For this review, take the finished solid that the model builds, in its own axes (mm). Face numbers are marked on the shaded views. A direction names the side the tool comes from. Give positions to 0.01 mm unless a question says otherwise; leave off trailing zeros. Write each loop counter-clockwise with the first axis right and the second up, starting at its lowest first coordinate (ties: lowest second). Pieces come first, ordered by that corner, then holes. Notation, with made-up numbers: M 88,73 L 102,73 A14 ccw 102,98 Z; hole C 30,-7.5 d1. An arc over 180 degrees is marked long. Write item = value, one per line.
Autodesk Inventor part; units mm, degrees
ref_plane "Work Plane1" through (0.5, 0, 0) normal (0, 0, -1) x (1, 0, 0)
ref_plane "YZ Plane" through (0, 0, 0) normal (1, 0, 0) x (0, 1, 0)
ref_plane "XZ Plane" through (0, 0, 0) normal (0, 1, 0) x (-1, 0, 0)
sketch "草图1" plane through (0, 0, 0) normal (0, 0, 1) x (1, 0, 0)
  line L0 (-0.580263, 0) -> (3.481577, 0)
  line L1 (0, 3.8) -> (0, 13.95)
  line L2 (0, 20.221695) -> (2.694468, 26)
  line L3 (2.694468, 26) -> (3.600776, 25.577382)
  line L4 (3.600776, 25.577382) -> (1, 20)
  line L5 (1, 20) -> (1, 15.25)
  line L6 (1, 15.25) -> (0, 15.25)
  dimension "d1" = 1
  dimension "d2" = 30.5
  dimension "d3" = 40
  dimension "d4" = 52
  dimension "d5" = 25
  dimension "d6" = 1
sketch "草图1 outline for 轴承体" plane through (0, 0, 0) normal (0, 0, 1) x (1, 0, 0)
  line L0 (2.694468, 26) -> (0, 20.221695)
  line L1 (3.600776, 25.577382) -> (2.694468, 26)
  line L2 (1, 20) -> (3.600776, 25.577382)
  line L3 (1, 15.25) -> (1, 20)
  line L4 (0, 15.25) -> (1, 15.25)
  line L5 (0, 20.221695) -> (0, 15.25)
revolve "轴承体" add sketch "草图1 outline for 轴承体" angle 360 about axis through (-10, 0, 0) along (1, 0, 0)
sketch "草图2" plane through (0, 0, 0) normal (-1, 0, 0) x (0, 0, 1)
  line L0 (0, -36.4) -> (0, 36.4)
  line L1 (2.4, 15.059963) -> (2.4, 11.75)
  line L2 (2.4, 11.75) -> (0, 11.75)
  line L3 (-2.4, 15.059963) -> (-2.4, 11.75)
  line L4 (-2.4, 11.75) -> (0, 11.75)
  line L5 (-36.4, 0) -> (36.4, 0)
  circle A0 centre (0, 0) radius 15.25
  circle A1 centre (0, 0) radius 26
  circle A2 centre (0, 0) radius 20
  line L6 (-2.4, 12.75) -> (2.4, 12.75)
  circle A3 centre (0, 0) radius 20.221695
  line L7 (2.4, 19.855478) -> (2.4, 25.888994)
  line L8 (0, 36.4) -> (0, -36.4)
  line L9 (0, 0) -> (13, 22.51666) construction
  line L10 (7.849278, 18.395348) -> (10.866036, 23.620526)
  line L11 (12.0062, 15.995348) -> (15.022958, 21.220526)
  line L12 (-2.4, 19.855478) -> (-2.4, 25.888994)
  line L13 (0, 0) -> (22.51666, 13) construction
  line L14 (15.995348, 12.0062) -> (21.220526, 15.022958)
  line L15 (18.395348, 7.849278) -> (23.620526, 10.866036)
  line L16 (0, 0) -> (-25.114071, -6.729295) construction
  line L17 (-19.800085, -2.820754) -> (-25.628013, -4.382343)
  line L18 (-18.557753, -7.457198) -> (-24.385682, -9.018787)
  line L19 (0, 0) -> (-18.384776, -18.384776) construction
  line L20 (0, 0) -> (-6.729295, -25.114071) construction
  line L21 (-15.736999, -12.342887) -> (-20.003339, -16.609227)
  line L22 (-12.342887, -15.736999) -> (-16.609227, -20.003339)
  line L23 (-7.457198, -18.557753) -> (-9.018787, -24.385682)
  line L24 (-2.820754, -19.800085) -> (-4.382343, -25.628013)
  dimension "d9" = 4.8
  dimension "d21" = 1
  dimension "d25" = 27
  dimension "d32" = 4.8
  dimension "d34" = 4.8
  dimension "d36" = 30
  dimension "d38" = 2.4
  dimension "d39" = 30
  dimension "d40" = 15
  dimension "d41" = 4.8
  dimension "d42" = 30
  dimension "d43" = 30
  dimension "d45" = 4.8
  dimension "d47" = 4.8
sketch "草图2 outline for 切口" plane through (0, 0, 0) normal (-1, 0, 0) x (0, 0, 1)
  arc A0 (-7.457198, -18.557753) -> (-12.342887, -15.736999) centre (0, 0) cw
  line L0 (-9.018787, -24.385682) -> (-7.457198, -18.557753)
  arc A1 (-16.609227, -20.003339) -> (-9.018787, -24.385682) centre (0, 0) ccw
  line L1 (-12.342887, -15.736999) -> (-16.609227, -20.003339)
  arc A2 (-15.736999, -12.342887) -> (-18.557753, -7.457198) centre (0, 0) cw
  line L2 (-20.003339, -16.609227) -> (-15.736999, -12.342887)
  arc A3 (-24.385682, -9.018787) -> (-20.003339, -16.609227) centre (0, 0) ccw
  line L3 (-18.557753, -7.457198) -> (-24.385682, -9.018787)
  line L4 (2.4, 25.888994) -> (2.4, 19.855478)
  arc A4 (10.866036, 23.620526) -> (2.4, 25.888994) centre (0, 0) ccw
  line L5 (7.849278, 18.395348) -> (10.866036, 23.620526)
  arc A5 (2.4, 19.855478) -> (7.849278, 18.395348) centre (0, 0) cw
  line L6 (15.022958, 21.220526) -> (12.0062, 15.995348)
  arc A6 (21.220526, 15.022958) -> (15.022958, 21.220526) centre (0, 0) ccw
  line L7 (15.995348, 12.0062) -> (21.220526, 15.022958)
  arc A7 (12.0062, 15.995348) -> (15.995348, 12.0062) centre (0, 0) cw
  arc A8 (-19.800085, -2.820754) -> (-2.4, 19.855478) centre (0, 0) cw
  line L8 (-25.628013, -4.382343) -> (-19.800085, -2.820754)
  arc A9 (-2.4, 25.888994) -> (-25.628013, -4.382343) centre (0, 0) ccw
  line L9 (-2.4, 19.855478) -> (-2.4, 25.888994)
  line L10 (23.620526, 10.866036) -> (18.395348, 7.849278)
  arc A10 (-4.382343, -25.628013) -> (23.620526, 10.866036) centre (0, 0) ccw
  line L11 (-2.820754, -19.800085) -> (-4.382343, -25.628013)
  arc A11 (18.395348, 7.849278) -> (-2.820754, -19.800085) centre (0, 0) cw
extrude "切口" cut sketch "草图2 outline for 切口" against normal through all
extrude "榫1" add sketch "草图2" against normal blind 1 contours L4 L3 L6 L0 | L0 L6 L1 L2 | A0 L0 L6 L3 | L1 L6 L0 A0
extrude "榫2" add sketch "草图2" against normal blind 5 contours L4 L3 L6 L0 | L0 L6 L1 L2
ref_plane "Work Plane1" through (0.5, 0, 0) normal (0, 0, -1) x (1, 0, 0)
equation "\"d1\" = SD"
equation "\"d2\" = SD1"
equation "\"d3\" = LADI"
equation "\"d4\" = SD2"
equation "\"d5\" = FAWI"
equation "\"d6\" = SD"
equation "\"d9\" = TW0"
equation "\"d21\" = SD"
equation "\"d25\" = SD3"
equation "\"d32\" = TW0"
equation "\"d34\" = TW0"
equation "\"d36\" = SEWI"
equation "\"d39\" = SEWI"
equation "\"d40\" = ANG1"
equation "\"d41\" = TW0"
equation "\"d42\" = SEWI"
equation "\"d43\" = SEWI"
equation "\"d45\" = TW0"
equation "\"d47\" = TW0"
equation "\"d17\" = SD"
equation "\"d13\" = SD"
equation "\"d23\" = TL1"
equation "\"FAWI\" = 25deg"
equation "\"SD1\" = 30.5"
equation "\"SD2\" = 52"
equation "\"SD\" = 1"
equation "\"TW0\" = 4.8"
equation "\"LADI\" = 40"
equation "\"d8\" = SD1"
equation "\"TL1\" = 5"
equation "\"SD3\" = 27"
equation "\"SEWI\" = 30deg"
equation "\"ANG1\" = 15deg"
equation "\"RR\" = 0.1"
equation "\"PB\" = TW0"
equation "\"PNT\" = TL1"
properties part number "垫圈 GB 858 30" material "钢，软"
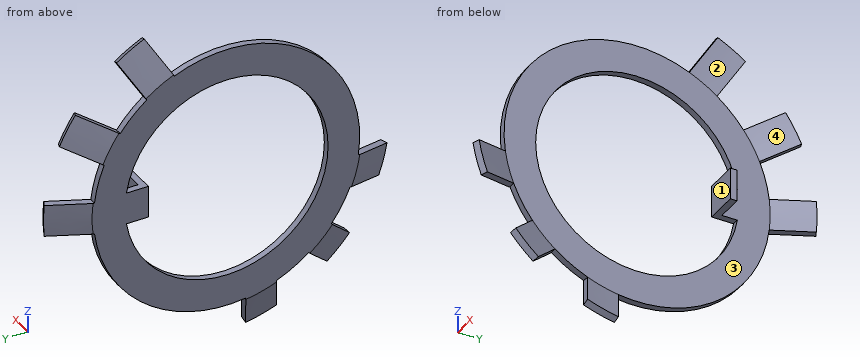
1. We need section B-B, the plane y = 0. Write out the cut boundary in (x, z).
Responses:
outline = M 0,-20 L 1,-20 L 1,-15.25 L 0,-15.25 Z; M 0,15.25 L 1,15.25 L 1,20 L 0,20 Z
2. We need section A-A, the plane z = 0. Write out the cut boundary in (x, y).
Responses:
outline = M 0,-20 L 1,-20 L 1,-15.25 L 0,-15.25 Z; M 0,11.75 L 5,11.75 L 5,12.75 L 1,12.75 L 1,20 L 3.6,25.58 L 2.69,26 L 0,20.22 Z
3. Insertion check: P1, Ø12, axis at y = -3, z = 7, coming from the +X side; P2, Ø12, axis at y = 9.5, z = -0.5, coming from the +X side; P3, Ø1.1, axis at x = 1, y = 22.5, coming from the +Z side; P4, Ø2.5, axis at x = 2.5, y = 14, coming from the +Z side. Each pin has a flat end and moves straight along its axis. Give the tip position at first contact, or say it passes through.
Responses:
P1 = through
P2 = 5
P3 = 2.4
P4 = 22.65
4. Machinability: for the marked faces 1, 2, 3 and 4, which of the approach directions +Z, -Z, +X, -X, +Y, -Y give a long, thin tool a straight path to every point of the face, cutting with its end or side? Answer none if there is none.
Responses:
face_1 = +X, -X
face_2 = +X, -Y
face_3 = +X
face_4 = -Z, +X, -Y
5. We need section C-C, the plane z = -10.5. Write out the cut boundary in (x, y).
Responses:
outline = M 0,-17.02 L 1,-17.02 L 1,-11.06 L 0,-11.06 Z; M 0,11.06 L 1,11.06 L 1,17.02 L 0,17.02 Z
6. For line 1 along Z through (x, y) = (0.4, 0); line 2 along Z through (x, y) = (1.3, 22); line 3 along Y through (x, z) = (0.65, 0), list the stretches that pass through material, from the lowest coordinate up. Write a range as from..to.
Responses:
line_1 = -20..-15.25, 15.25..20
line_2 = -2.4..2.4
line_3 = -20..-15.25, 11.75..21.62
